Autodesk Fusion 360 part; units mm, degrees
sketch "Sketch1" plane through (0, 0, 0) normal (0, 0, 1) x (1, 0, 0)
  circle A0 centre (0, 0) radius 8.75
  dimension "d1" = 17.5
extrude "Extrude1" add sketch "Sketch1" along normal blind 2
sketch "Sketch2" plane through (0, 0, 2) normal (0, 0, 1) x (-1, 0, 0)
  circle A0 centre (0, 0) radius 8.75
  circle A1 centre (0, 0) radius 5
  dimension "d4" = 10
extrude "Extrude2" add sketch "Sketch2" along normal blind 25 contours A1
sketch "Sketch3" plane through (0, 0, 0) normal (0, 0, -1) x (1, 0, 0)
  circle A0 centre (0, 0) radius 8.75
  circle A1 centre (0, 0) radius 3.75
  dimension "d7" = 7.5
extrude "Extrude3" cut sketch "Sketch3" against normal blind 26 contours A1
sketch "Sketch4" plane through (0, 0, 0) normal (0, 0, 1) x (1, 0, 0)
sketch "Sketch5" plane through (0, 0, 0) normal (1, 0, 0) x (0, 1, 0)
  line L0 (-3.75, 26) -> (3.75, 26)
  line L1 (3.75, 26) -> (3.75, 16)
  line L2 (3.75, 16) -> (-3.75, 16)
  line L3 (-3.75, 16) -> (-3.75, 26)
  dimension "d10" = 7.5
  dimension "d11" = 10
extrude "Extrude4" add sketch "Sketch5" along normal mid plane 1
Geometry check sheet. Reference: the model listing, model coordinates, mm. A direction names the side the tool comes from. Coordinates: 2 decimals unless noted, no trailing zeros. Order: outer loops, then holes, each group sorted by start corner. A loop starts at its lowest first (then second) coordinate and runs counter-clockwise, first axis right, second up. Notation, with made-up numbers: (9, 16) -> (53, 16) arc R26 cw to (53, 38) -> close; hole circle Ø8 at (50.25, -40). An arc over 180 degrees is marked (long way). Use a Markdown table: item, result. Add a question column.
1. Material ranges on L1, parallel to X at y = 0, z = 16.5; L2, parallel to Y at x = 0, z = 6, recorded low to high.
2. Mould release check, pull along X, two halves, no side actions. Record for faces 1 (the face through (-6.944, 5.324, 0.986)), 2 (the face through (0.5, 0, 21)), 3 (the face through (0, -4, 0)): pulls with the +X half, pulls with the -X half, needs draft (parallel to the pull), parting line crosses it, or undercut.
3. Cross-section at A-A (y = 0). Enter the section's corners in (x, z).
4. Cross-section at D-D (z = 3). Enter the section's corners in (x, y).
5. Set-up check for faces 4 (the face through (0, 0, 27)), 5 (the face through (2, 0, 26)), 6 (the face through (4, -4, 2)): record each of +Z, -Z, +X, -X, +Y, -Y from which the full face is reachable in a straight line by a thin tool's end or side.
6. Cross-section at B-B (z = 21.25). Enter the section's corners in (x, y).
7. Go/stop test with flat-tipped pins: pin 1 Ø3.5 at (y, z) = (1.5, 21.5) entering from +X; pin 2 Ø5 at (x, y) = (3, -2.5) entering from -Z; pin 3 Ø4 at (x, z) = (-3, 6.5) entering from +Y; pin 4 Ø1.6 at (x, y) = (-1.5, -1.5) entering from -Z. Record where each tip stops, or that it passes through.
8. Cross-section at C-C (x = 0). Enter the section's corners in (y, z), and give its area (3 significant figures).
Filled sheet:
| question | item | result |
|---|---|---|
| 1 | L1 | -5 to -3.75, -0.5 to 0.5, 3.75 to 5 |
| 1 | L2 | -5 to -3.75, 3.75 to 5 |
| 2 | face 1 | parting line crosses it |
| 2 | face 2 | undercut |
| 2 | face 3 | needs draft |
| 3 | outline | (-8.75, 0) -> (-3.75, 0) -> (-3.75, 26) -> (-0.5, 26) -> (-0.5, 16) -> (0.5, 16) -> (0.5, 26) -> (3.75, 26) -> (3.75, 0) -> (8.75, 0) -> (8.75, 2) -> (5, 2) -> (5, 27) -> (-5, 27) -> (-5, 2) -> (-8.75, 2) -> close |
| 4 | outline | circle Ø10 at (0, 0); hole circle Ø7.5 at (0, 0) |
| 5 | face 4 | +Z, +X, -X, +Y, -Y |
| 5 | face 5 | -Z |
| 5 | face 6 | +Z |
| 6 | outline | circle Ø10 at (0, 0); hole (-0.5, -3.72) -> (-0.5, 3.72) arc R3.75 ccw to start; hole (0.5, -3.72) arc R3.75 ccw to (0.5, 3.72) -> close |
| 7 | pin 1 | x = 5 |
| 7 | pin 2 | z = 0 |
| 7 | pin 3 | y = 4.9 |
| 7 | pin 4 | z = 26 |
| 8 | outline | (-8.75, 0) -> (-3.75, 0) -> (-3.75, 16) -> (3.75, 16) -> (3.75, 0) -> (8.75, 0) -> (8.75, 2) -> (5, 2) -> (5, 27) -> (-5, 27) -> (-5, 2) -> (-8.75, 2) -> close |
| 8 | area | 165 mm2 |
